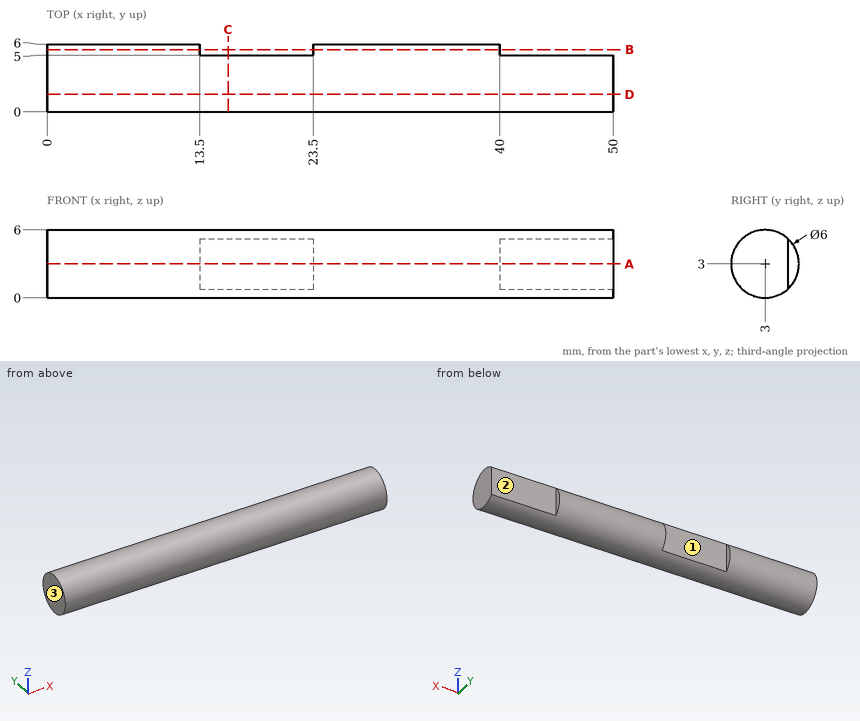
Part print with two shaded views. Sizes in mm from the minimum x, y, z corner. A direction names the side the tool comes from. Round coordinates to 2 decimals unless told otherwise and drop trailing zeros. Order: outer loops, then holes, each group sorted by start corner. A loop starts at its lowest first (then second) coordinate and runs counter-clockwise, first axis right, second up. Notation, with made-up numbers: M 55.25,-31 L 87.25,-31 A30 ccw 87.25,2 Z; hole C 64.25,20.5 d1. An arc over 180 degrees is marked long. Answer in a Markdown table with one row per item. Add a question column.
Q1. Cut at B-B on y = 5.5. Give the cut face in (x, z).
Q2. Cut at C-C on x = 16. Give the cut face in (y, z).
Q3. Cut at A-A on z = 3. Give the cut face in (x, y).
Q4. Pin check, flat tips, straight feed: pin 1 (0.8 mm diameter, centred on y = 5.5, z = 2, fed in from +X); pin 2 (1.3 mm diameter, centred on x = 45.5, z = 2.5, fed in from +Y); pin 3 (1.5 mm diameter, centred on x = 27.5, y = 5, fed in from -Z). Stop position of each tip, or through.
Q5. Cut at D-D on y = 1.55. Give the cut face in (x, z).
Q6. 3-axis set-ups, long thin cutter, end or side, ignore diameter. For the marked faces 1, 2 and 3: which of +Z, -Z, +X, -X, +Y, -Y reach the whole face in a straight line?
Q7. Wall check: L1, parallel to Z at x = 31, y = 2.8; L2, parallel to Y at x = 5, z = 4.7; L3, parallel to Z at x = 35.5, y = 0.95. Give the ranges that are in metal, low to high. Write a range as from..to.
Established:
| question | item | result |
|---|---|---|
| 1 | outline | M 0,1.34 L 13.5,1.34 L 13.5,4.66 L 0,4.66 Z; M 23.5,1.34 L 40,1.34 L 40,4.66 L 23.5,4.66 Z |
| 2 | outline | M 5,0.76 L 5,5.24 A3 ccw long Z |
| 3 | outline | M 0,0 L 50,0 L 50,5 L 40,5 L 40,6 L 23.5,6 L 23.5,5 L 13.5,5 L 13.5,6 L 0,6 Z |
| 4 | pin 1 | stops at x = 40 |
| 4 | pin 2 | stops at y = 5 |
| 4 | pin 3 | stops at z = 0.27 |
| 5 | outline | M 0,0.37 L 50,0.37 L 50,5.63 L 0,5.63 Z |
| 6 | face 1 | +Z, -Z, +Y |
| 6 | face 2 | +Z, -Z, +X, +Y |
| 6 | face 3 | +Z, -Z, -X, +Y, -Y |
| 7 | L1 | z = 0.01..5.99 |
| 7 | L2 | y = 0.53..5.47 |
| 7 | L3 | z = 0.81..5.19 |
